Check sheet for the drawn part. Datum: minimum x, y, z corner. Units: mm. A direction names the side the tool comes from. Give positions to 0.01 mm unless a question says otherwise; leave off trailing zeros. Write each loop counter-clockwise with the first axis right and the second up, starting at its lowest first coordinate (ties: lowest second). Pieces come first, ordered by that corner, then holes.
(1) Cross-section at B-B (y = 15). Record the boundary of the cut face in (x, z).
(2) Cross-section at D-D (x = 7.5). Record the boundary of the cut face in (y, z), and give its area (3 significant figures).
(3) Thickness scan on line 1 along Z through (x, y) = (5, 1.5); line 2 along Z through (x, y) = (7.25, 11.5); line 3 along Y through (x, z) = (5, 1.65). Record the ranges inside material, lowest first.
(4) Depth check by flat-ended pin: P1, Ø2, axis at x = 3, z = 8, coming from the +Y side; P2, Ø1.5, axis at x = 1, z = 2.5, coming from the -Y side; P3, Ø5, axis at x = 6, y = 11, coming from the +Z side; P4, Ø1, axis at y = 9, z = 4, coming from the +X side. Enter the tip coordinate at first touch or a pass-through.
(5) Tool access check on the marked faces 1 and 2. Record the directions out of +Z, -Z, +X, -X, +Y, -Y that give a thin tool (end or side, any length) a straight path to the whole face; none if there is none.
(6) Mould release check, pull along Y, two halves, no side actions. Record for the marked faces 3, 4, 5 and 6: +Y half, -Y half, draft (parallel to the pull), parting line (faces both ways), or undercut.
(7) Cross-section at A-A (z = 7). Record the boundary of the cut face in (x, y).
(8) Cross-section at C-C (x = 5). Record the boundary of the cut face in (y, z).
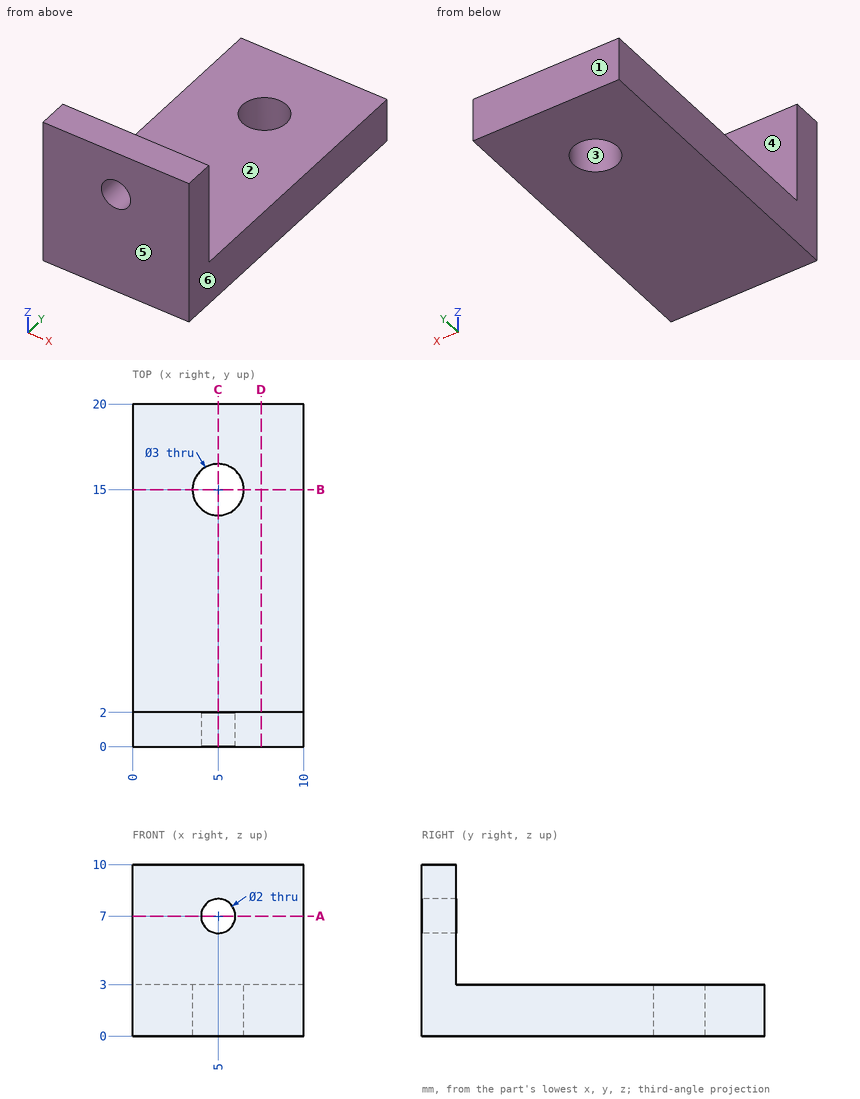
Reply:
1. outline: (0, 0) - (3.5, 0) - (3.5, 3) - (0, 3) - close; (6.5, 0) - (10, 0) - (10, 3) - (6.5, 3) - close
2. outline: (0, 0) - (20, 0) - (20, 3) - (2, 3) - (2, 10) - (0, 10) - close
2. area: 74.0 mm2
3. line 1: z = 0 to 6, 8 to 10
3. line 2: z = 0 to 3
3. line 3: y = 0 to 13.5, 16.5 to 20
4. P1: stops at y = 2
4. P2: stops at y = 0
4. P3: stops at z = 3
4. P4: passes through
5. face 1: +Z, -Z, +X, -X, +Y
5. face 2: +Z, +X, -X, +Y
6. face 3: undercut
6. face 4: +Y half
6. face 5: -Y half
6. face 6: draft
7. outline: (0, 0) - (4, 0) - (4, 2) - (0, 2) - close; (6, 0) - (10, 0) - (10, 2) - (6, 2) - close
8. outline: (0, 0) - (13.5, 0) - (13.5, 3) - (2, 3) - (2, 6) - (0, 6) - close; (0, 8) - (2, 8) - (2, 10) - (0, 10) - close; (16.5, 0) - (20, 0) - (20, 3) - (16.5, 3) - close
